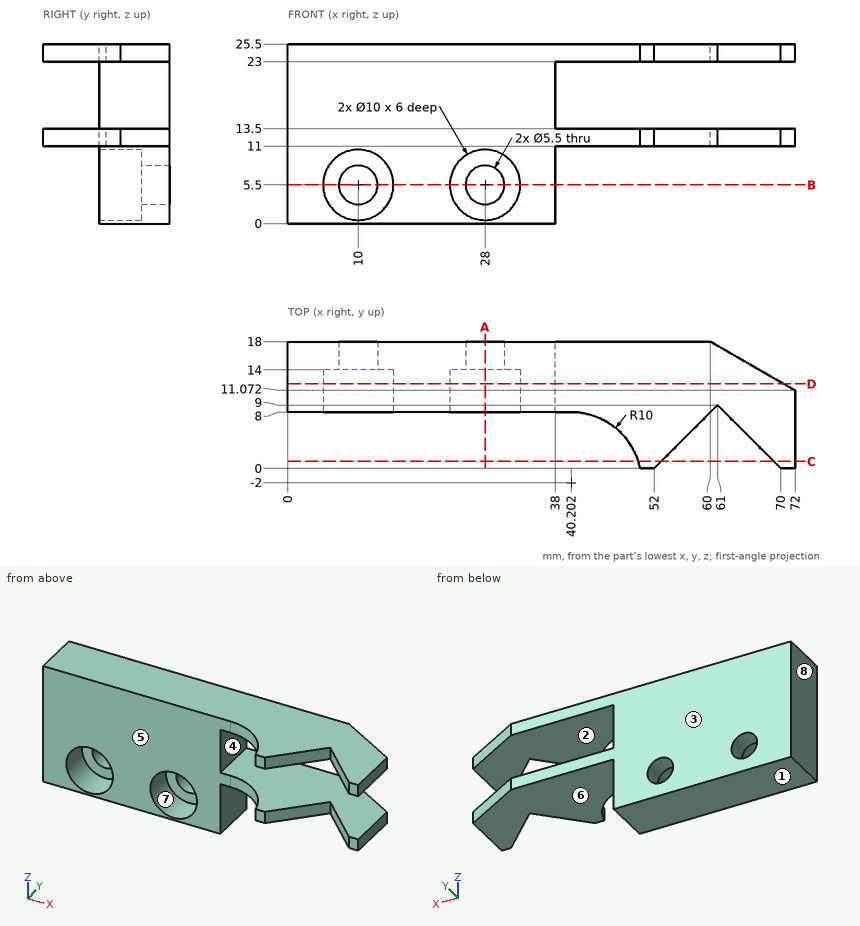
Could you check a few things on this drawing? It's one solid part, dimensions in mm from its lowest x, y, z. A direction names the side the tool comes from. Give positions to 0.01 mm unless a question says otherwise; leave off trailing zeros. Write each loop counter-clockwise with the first axis right and the second up, starting at its lowest first coordinate (ties: lowest second). Pieces come first, ordered by that corner, then holes. Notation, with made-up numbers: (-38.5, -27) -> (8.5, -27) arc R4 cw to (8.5, -21) -> close; hole circle Ø5 at (79, 49.25). An arc over 180 degrees is marked (long way). Answer as CSV lines item,"result". Start each with the question number.
(1) If we section it at D-D, the plane y = 12: Write out the boundary of the cut face in (x, z), and give its area (3 significant figures).
(2) If we section it at B-B, the plane z = 5.5: Write out the boundary of the cut face in (x, y).
(3) If we section it at C-C, the plane y = 1: Write out the boundary of the cut face in (x, z), and give its area (3 significant figures).
(4) Please list where these lines run through material, in increasing order: line 1 (X direction, y = 12.5, z = 5.5); line 2 (X direction, y = 16.75, z = 5.5); line 3 (Z direction, x = 54.5, y = 8.25).
(5) If we mould it in two halves opening along Z, with no side actions, what happens to the marked faces 1, 2 and 3? For each: +Z half, -Z half, draft (parallel to the pull), parting line (faces both ways), or undercut.
(6) I'm going to push flat-ended pins straight in: pin 1 Ø10 at (x, y) = (46.5, 4) entering from -Z; pin 2 Ø1.5 at (x, z) = (31.5, 18) entering from -Y; pin 3 Ø5 at (y, z) = (11.5, 3) entering from +X. Where does each tip first touch, or does it pass through?
(7) Which directions (+Z, -Z, +X, -X, +Y, -Y) give clear straight access to the entire face, cutting with the end or side of a thin tool? Please do the marked faces 4, 5, 6, 7 and 8.
(8) If we section it at A-A, the plane x = 28: Write out the boundary of the cut face in (y, z), and give its area (3 significant figures).
Answer list:
1,outline,"(0, 0) -> (38, 0) -> (38, 11) -> (70.39, 11) -> (70.39, 13.5) -> (38, 13.5) -> (38, 23) -> (70.39, 23) -> (70.39, 25.5) -> (0, 25.5) -> close; hole circle Ø10 at (10, 5.5); hole circle Ø10 at (28, 5.5)"
1,area,"974 mm^2"
2,outline,"(0, 8) -> (5, 8) -> (5, 14) -> (7.25, 14) -> (7.25, 18) -> (0, 18) -> close; (12.75, 14) -> (15, 14) -> (15, 8) -> (23, 8) -> (23, 14) -> (25.25, 14) -> (25.25, 18) -> (12.75, 18) -> close; (30.75, 14) -> (33, 14) -> (33, 8) -> (38, 8) -> (38, 18) -> (30.75, 18) -> close"
3,outline,"(49.74, 11) -> (53, 11) -> (53, 13.5) -> (49.74, 13.5) -> close; (49.74, 23) -> (53, 23) -> (53, 25.5) -> (49.74, 25.5) -> close; (69, 11) -> (72, 11) -> (72, 13.5) -> (69, 13.5) -> close; (69, 23) -> (72, 23) -> (72, 25.5) -> (69, 25.5) -> close"
3,area,"31.3 mm^2"
4,line 1,"0 to 5, 15 to 23, 33 to 38"
4,line 2,"0 to 7.25, 12.75 to 25.25, 30.75 to 38"
4,line 3,"11 to 13.5, 23 to 25.5"
5,face 1,"-Z half"
5,face 2,"undercut"
5,face 3,"draft"
6,pin 1,"z = 11"
6,pin 2,"y = 8"
6,pin 3,"x = 38"
7,face 4,"+X, +Y, -Y"
7,face 5,"+Z, -Z, -X, -Y"
7,face 6,"-Z, +X, +Y, -Y"
7,face 7,"-Y"
7,face 8,"+Z, -Z, -X, +Y, -Y"
8,outline,"(8, 0) -> (18, 0) -> (18, 2.75) -> (14, 2.75) -> (14, 0.5) -> (8, 0.5) -> close; (8, 10.5) -> (14, 10.5) -> (14, 8.25) -> (18, 8.25) -> (18, 25.5) -> (8, 25.5) -> close"
8,area,"173 mm^2"
